from build123d import *

# Parameters (mm, degrees)
BOSS_EXTRUDE1_DEPTH = 2.54
SKETCH2_R           = 2.032
CUT_EXTRUDE1_DEPTH  = 120.845185189
FILLET1_R           = 12.7


with BuildPart() as part:
    # Sketch1 → Boss-Extrude1 (new body)
    with BuildSketch(Plane(origin=(0, 0, 0), x_dir=(0, 0, -1), z_dir=(1, 0, 0))):
        with BuildLine():
            Line((-25.711264461, 93.961261583), (-9.389037217, -1.603622507))
            ThreePointArc((-9.389037217, -1.603622507), (1.603622507, -9.389037217), (9.389037217, 1.603622507))
            Line((9.389037217, 1.603622507), (4.740879345, 28.818086661))
            ThreePointArc((4.740879345, 28.818086661), (4.758501249, 33.195142409), (6.261073005, 37.306250004))
            Line((6.261073005, 37.306250004), (21.384041616, 63.5))
            ThreePointArc((21.384041616, 63.5), (32.382564244, 69.85), (43.381086873, 63.5))
            Line((43.381086873, 63.5), (51.629978844, 49.2125))
            ThreePointArc((51.629978844, 49.2125), (55.658330241, 47.893886054), (57.407660819, 51.754740913))
            Line((57.407660819, 51.754740913), (47.914524724, 81.863122013))
            Line((47.914524724, 81.863122013), (-13.005337503, 104.493706378))
            ThreePointArc((-13.005337503, 104.493706378), (-22.400947675, 102.898013226), (-25.711264461, 93.961261583))
        make_face()
    extrude(amount=BOSS_EXTRUDE1_DEPTH)

    # Sketch2 → Cut-Extrude1 (cut, through all)
    with BuildSketch(Plane(origin=(2.54, 0, 0), x_dir=(0, 0, -1), z_dir=(1, 0, 0))):
        Circle(SKETCH2_R)
        with Locations((-16.322227244, 95.56488409)):
            Circle(SKETCH2_R)
    extrude(amount=-CUT_EXTRUDE1_DEPTH, mode=Mode.SUBTRACT)

    # Fillet1
    fillet1_edges = [part.edges().sort_by_distance(p)[0] for p in [
        (1.27, 81.863122013, -47.914524724),
    ]]
    fillet(fillet1_edges, radius=FILLET1_R)


solid = part.part
Read the model definition and answer for the solid it produces. Units are mm, in the model's axes. A direction names the side the tool comes from. Round coordinates to 2 decimals unless told otherwise and drop trailing zeros. Write each loop counter-clockwise with the first axis right and the second up, starting at its lowest first coordinate (ties: lowest second). Pieces come first, ordered by that corner, then holes.
1. Given pin 1 Ø1 at (x, z) = (1.5, -18.5) entering from -Y; pin 2 Ø1.5 at (x, z) = (2, -9) entering from +Y, each flat-ended and moving along its own axis, determine where each tip first touches the part or whether it passes through.
2. The part is cut by section B-B, the plane x = 0.55. State how many separate pieces and enclosed holes the cut face has, then the cut area to 3 significant figures.
3. Straight lines are drawn through the part: L1, parallel to Z at x = 1.5, y = 65; L2, parallel to Y at x = 1.35, z = 0 (3 decimals); L3, parallel to Z at x = 1.95, y = 1.5. For each, find the intervals that lie inside material, in ascending order.
4. The part is cut by section C-C, the plane y = 0. Determine the outline of the cut face in (x, z) (3 decimals).
5. Determine the mould class of faces 4 (the face through (1.252, 33.134, -4.748)), 5 (the face through (1.252, 56.456, -47.448)), 6 (the face through (1.29, 80.93, -46.82)) for opening direction Y: pulls with the +Y half, pulls with the -Y half, needs draft (parallel to the pull), parting line crosses it, or undercut.
6. The part is cut by section D-D, the plane y = 89. Determine the outline of the cut face in (x, z), then the cut area to 3 significant figures.
7. The part is cut by section A-A, the plane z = 0. Determine the outline of the cut face in (x, y) (3 decimals).
8. Which of the six approach directions +Z, -Z, +X, -X, +Y, -Y give full straight-line access (tool end or side, diameter ignored) to faces 1 (the face through (1.3, 15, -7.1)), 2 (the face through (2.54, 61, -6)), 3 (the face through (1.252, 50.22, -13.717))?
Values:
1. pin 1: stops at y = 57.64
1. pin 2: stops at y = 96.6
2. separate pieces: 1
2. enclosed holes: 2
2. area: 4,000 mm2
3. L1: z = -53.23 to -42.37, -22.4 to 20.76
3. L2: y = -9.525 to -2.032, 2.032 to 99.662
3. L3: z = -9.41 to -1.37, 1.37 to 9.92
4. outline: (0, -9.525) - (2.54, -9.525) - (2.54, -2.032) - (0, -2.032) - close; (0, 2.032) - (2.54, 2.032) - (2.54, 9.663) - (0, 9.663) - close
5. face 4: undercut
5. face 5: pulls with the -Y half
5. face 6: pulls with the +Y half
6. outline: (0, -28.7) - (2.54, -28.7) - (2.54, 24.86) - (0, 24.86) - close
6. area: 136 mm2
7. outline: (0, -9.525) - (2.54, -9.525) - (2.54, -2.032) - (0, -2.032) - close; (0, 2.032) - (2.54, 2.032) - (2.54, 99.662) - (0, 99.662) - close
8. face 1: -Z, +X, -X
8. face 2: +Z, -Z, +X, +Y, -Y
8. face 3: +X, -X
